```python
from build123d import *

# Parameters (mm, degrees)
SKETCH1_R           = 0.925
SKETCH1_R_2         = 0.92499942
BOSS_EXTRUDE1_DEPTH = 1.041


with BuildPart() as part:
    # Sketch1 → Boss-Extrude1 (new body)
    with BuildSketch(Plane.XY):
        with BuildLine():
            Line((0, 5.75), (0, 0.635))
            ThreePointArc((0, 0.635), (0.185987194, 0.185987194), (0.635, 0))
            Line((0.635, 0), (28.321, 0))
            ThreePointArc((28.321, 0), (28.770012806, 0.185987194), (28.956, 0.635))
            Line((28.956, 0.635), (28.956, 5.53000114))
            ThreePointArc((28.956, 5.53000114), (28.706, 5.78000114), (28.956, 6.03000114))
            Line((28.956, 6.03000114), (28.956, 7.03000114))
            ThreePointArc((28.956, 7.03000114), (28.706, 7.28000114), (28.956, 7.53000114))
            Line((28.956, 7.53000114), (28.956, 8.53000114))
            ThreePointArc((28.956, 8.53000114), (28.706, 8.78000114), (28.956, 9.03000114))
            Line((28.956, 9.03000114), (28.956, 10.03000114))
            ThreePointArc((28.956, 10.03000114), (28.706, 10.28000114), (28.956, 10.53000114))
            Line((28.956, 10.53000114), (28.956, 11.53000114))
            ThreePointArc((28.956, 11.53000114), (28.706, 11.78000114), (28.956, 12.03000114))
            Line((28.956, 12.03000114), (28.956, 13.03000114))
            ThreePointArc((28.956, 13.03000114), (28.706, 13.28000114), (28.956, 13.53000114))
            Line((28.956, 13.53000114), (28.956, 14.53000114))
            ThreePointArc((28.956, 14.53000114), (28.706, 14.78000114), (28.956, 15.03000114))
            Line((28.956, 15.03000114), (28.956, 16.03000114))
            ThreePointArc((28.956, 16.03000114), (28.706, 16.28000114), (28.956, 16.53000114))
            Line((28.956, 16.53000114), (28.956, 17.53000114))
            ThreePointArc((28.956, 17.53000114), (28.706, 17.78000114), (28.956, 18.03000114))
            Line((28.956, 18.03000114), (28.956, 24.13))
            Line((28.956, 24.13), (26.416, 26.67))
            Line((26.416, 26.67), (0.635, 26.67))
            ThreePointArc((0.635, 26.67), (0.185987194, 26.484012806), (0, 26.035))
            Line((0, 26.035), (0, 18.25))
            ThreePointArc((0, 18.25), (0.25, 18), (0, 17.75))
            Line((0, 17.75), (0, 16.75))
            ThreePointArc((0, 16.75), (0.25, 16.5), (0, 16.25))
            Line((0, 16.25), (0, 15.25))
            ThreePointArc((0, 15.25), (0.25, 15), (0, 14.75))
            Line((0, 14.75), (0, 13.75))
            ThreePointArc((0, 13.75), (0.25, 13.5), (0, 13.25))
            Line((0, 13.25), (0, 12.25))
            ThreePointArc((0, 12.25), (0.25, 12), (0, 11.75))
            Line((0, 11.75), (0, 10.75))
            ThreePointArc((0, 10.75), (0.25, 10.5), (0, 10.25))
            Line((0, 10.25), (0, 9.25))
            ThreePointArc((0, 9.25), (0.25, 9), (0, 8.75))
            Line((0, 8.75), (0, 7.75))
            ThreePointArc((0, 7.75), (0.25, 7.5), (0, 7.25))
            Line((0, 7.25), (0, 6.25))
            ThreePointArc((0, 6.25), (0.25, 6), (0, 5.75))
        make_face()
        with Locations(Location((27.178, 3.683, 0), (0, 0, 180))):
            Circle(SKETCH1_R, mode=Mode.SUBTRACT)
        with Locations(Location((1.778, 3.683, 0), (0, 0, 180))):
            Circle(SKETCH1_R, mode=Mode.SUBTRACT)
        with Locations(Location((14.478, 21.59, 0), (0, 0, 180))):
            Circle(SKETCH1_R_2, mode=Mode.SUBTRACT)
    extrude(amount=-BOSS_EXTRUDE1_DEPTH)


solid = part.part
```
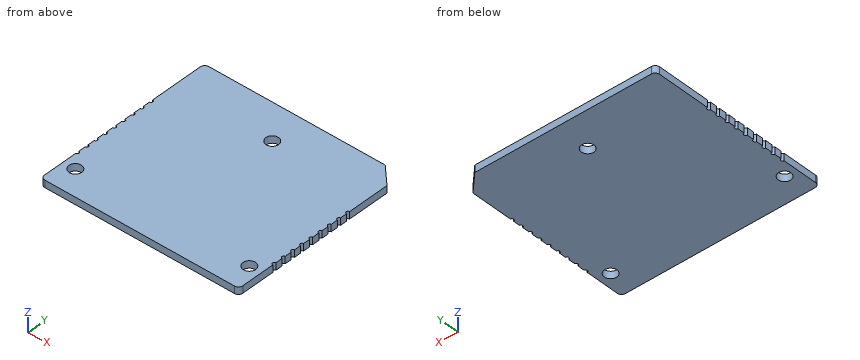
The listing builds one solid part. Answer for the finished solid, in the listing's coordinates (mm). Coordinates: 2 decimals unless noted, no trailing zeros. Loops run counter-clockwise (first coordinate to the right, second up) from the corner with the lowest first, then second, coordinate; pieces in that order, holes last. Notation, with made-up numbers: M 86.5,-25.75 L 134.5,-25.75 A15 cw 134.5,3.25 Z; hole C -24.75,19 d2. An arc over 180 degrees is marked long. Answer as a JSON object with one key per item and string values. Group by question number.
Item 1: Consider L1, parallel to X at y = 21.59, z = -0.5; L2, parallel to X at y = 4, z = -0.75; L3, parallel to Y at x = 28, z = -0.9. Determine where each line is inside the solid, lowest interval first.
Item 2: Section A-A (y = 21.59) is taken. Write down the section's boundary in (x, z), and give its area (3 significant figures).
Item 3: Section B-B (x = 2.25) is taken. Write down the section's boundary in (y, z).
Item 4: Section C-C (z = -0.8) is taken. Give the number of separate pieces and of enclosed holes in the cut face, and give its area (3 significant figures).
Solved:
{
 "1": {"L1": "x = 0 to 13.55, 15.4 to 28.96", "L2": "x = 0 to 0.91, 2.65 to 26.31, 28.05 to 28.96", "L3": "y = 0 to 3.26, 4.11 to 25.09"},
 "2": {"outline": "M 0,-1.04 L 13.55,-1.04 L 13.55,0 L 0,0 Z; M 15.4,-1.04 L 28.96,-1.04 L 28.96,0 L 15.4,0 Z", "area": "28.2 mm2"},
 "3": {"outline": "M 0,-1.04 L 2.89,-1.04 L 2.89,0 L 0,0 Z; M 4.48,-1.04 L 26.67,-1.04 L 26.67,0 L 4.48,0 Z"},
 "4": {"separate pieces": "1", "enclosed holes": "3", "area": "759 mm2"}
}
